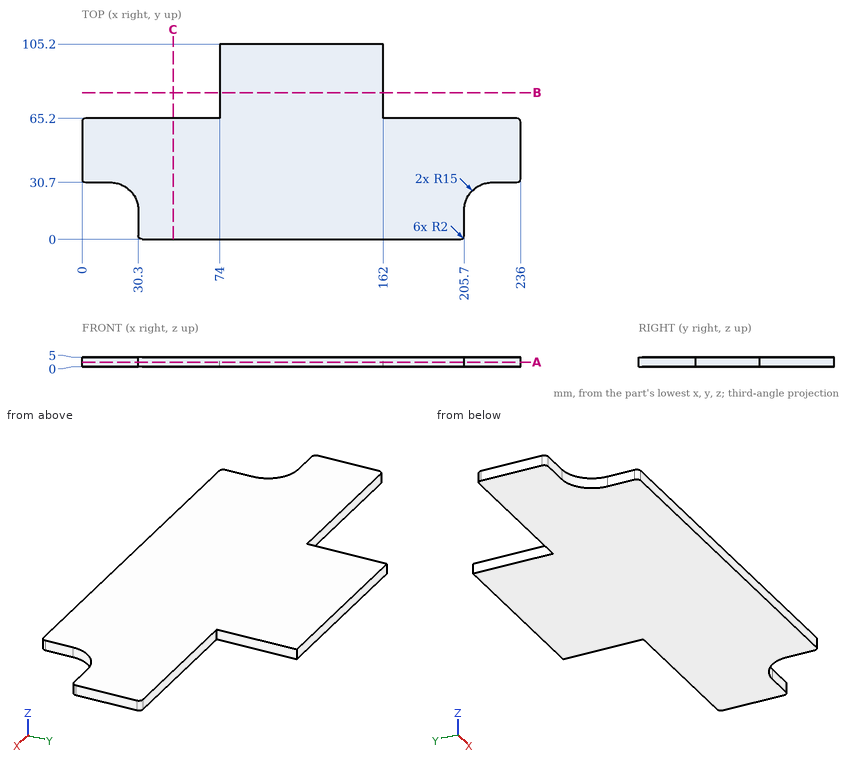
Geometry check sheet. Reference: drawing and pictorial views, mm from the part's lowest x, y, z. Coordinates: 2 decimals unless noted, no trailing zeros. Order: outer loops, then holes, each group sorted by start corner. A loop starts at its lowest first (then second) coordinate and runs counter-clockwise, first axis right, second up. Notation, with made-up numbers: (53, -7.5) -> (80, -7.5) arc R31 ccw to (80, 20.5) -> close; hole circle Ø4 at (88, -35). An arc over 180 degrees is marked (long way). Write item = value, one per line. Start each with the question number.
1) Cross-section at B-B (y = 79). Enter the section's corners in (x, z).
2) Cross-section at C-C (x = 49). Enter the section's corners in (y, z).
3) Go/stop test with flat-tipped pins: P1, Ø2.5, axis at y = 82, z = 2.5, coming from the +X side; P2, Ø1.5, axis at x = 32, z = 2.5, coming from the +Y side; P3, Ø1.5, axis at y = 66.5, z = 4, coming from the -X side. Record where each tip stops, or that it passes through.
4) Cross-section at A-A (z = 2.5). Enter the section's corners in (x, y), then the cut area to 3 significant figures.
5) Material ranges on L1, parallel to Y at x = 177.5, z = 2.45; L2, parallel to X at y = 9.5, z = 2.9; L3, parallel to X at y = 80.5, z = 0.3, recorded low to high.
Ans:
q1.outline = (74, 0) -> (162, 0) -> (162, 5) -> (74, 5) -> close
q2.outline = (0, 0) -> (65.2, 0) -> (65.2, 5) -> (0, 5) -> close
q3.P1 = 162
q3.P2 = 65.2
q3.P3 = 74
q4.outline = (0, 32.7) arc R2 ccw to (2, 30.7) -> (15.3, 30.7) arc R15 cw to (30.3, 15.7) -> (30.3, 2) arc R2 ccw to (32.3, 0) -> (203.7, 0) arc R2 ccw to (205.7, 2) -> (205.7, 15.7) arc R15 cw to (220.7, 30.7) -> (234, 30.7) arc R2 ccw to (236, 32.7) -> (236, 63.2) arc R2 ccw to (234, 65.2) -> (162, 65.2) -> (162, 105.2) -> (74, 105.2) -> (74, 65.2) -> (2, 65.2) arc R2 ccw to (0, 63.2) -> close
q4.area = 17,100 mm²
q5.L1 = 0 to 65.2
q5.L2 = 30.3 to 205.7
q5.L3 = 74 to 162
